Verification items for the finished model (mm, model axes). Face numbers are marked on the shaded views. A direction names the side the tool comes from. Round coordinates to 2 decimals unless told otherwise and drop trailing zeros. Write each loop counter-clockwise with the first axis right and the second up, starting at its lowest first coordinate (ties: lowest second). Pieces come first, ordered by that corner, then holes.
from build123d import *

# Parameters (mm, degrees)
EXTRUDE_1_DEPTH     = 34
SKETCH_2_R          = 2.75
CUT_EXTRUDE_1_DEPTH = 43.95346319
SKETCH_3_R          = 2.75
CUT_EXTRUDE_2_DEPTH = 45.226688775


with BuildPart() as part:
    # ｽｹｯﾁ1 → ﾎﾞｽ - 押し出し1 (new body)
    with BuildSketch(Plane.XY):
        Polygon((0, 0), (17, 0), (17, 17), (20, 17), (20, -3), (0, -3), align=None)
    extrude(amount=EXTRUDE_1_DEPTH)

    # ｽｹｯﾁ2 → ｶｯﾄ - 押し出し1 (cut, through all)
    with BuildSketch(Plane(origin=(20, 0, 0), x_dir=(0, 0, -1), z_dir=(1, 0, 0))):
        with Locations((-27, 7)):
            Circle(SKETCH_2_R)
        with Locations((-7, 7)):
            Circle(SKETCH_2_R)
    extrude(amount=-CUT_EXTRUDE_1_DEPTH, mode=Mode.SUBTRACT)

    # ｽｹｯﾁ3 → ｶｯﾄ - 押し出し2 (cut, through all)
    with BuildSketch(Plane.XZ.offset(3)):
        with Locations(Location((5, 7, 0), (0, 0, 270))):
            Circle(SKETCH_3_R)
        with Locations(Location((5, 27, 0), (0, 0, 270))):
            Circle(SKETCH_3_R)
    extrude(amount=-CUT_EXTRUDE_2_DEPTH, mode=Mode.SUBTRACT)


solid = part.part
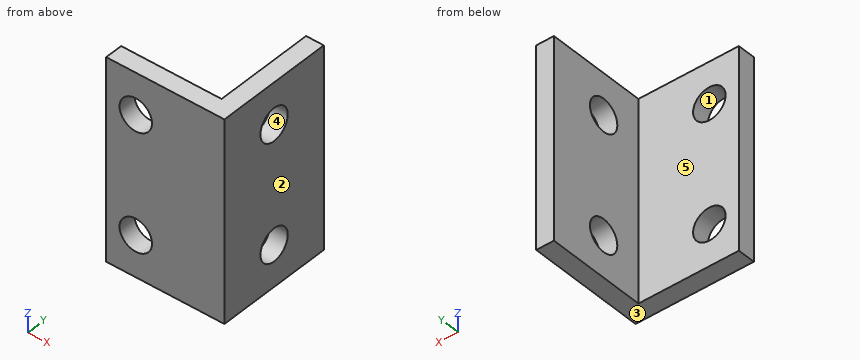
Q1. Material ranges on line 1 along Z through (x, y) = (7, -1.75); line 2 along X through (y, z) = (-2.15, 27); line 3 along X through (y, z) = (9, 11), recorded low to high.
Recorded:
line 1: z = 0 to 5.11, 8.89 to 25.11, 28.89 to 34
line 2: x = 0 to 2.25, 7.75 to 20
line 3: x = 17 to 20
Q2. Sectioned sample at A-A (y = 7). Enter the section's corners in (x, z).
Recorded:
outline: (17, 0) - (20, 0) - (20, 4.25) - (17, 4.25) - close; (17, 9.75) - (20, 9.75) - (20, 24.25) - (17, 24.25) - close; (17, 29.75) - (20, 29.75) - (20, 34) - (17, 34) - close
Q3. Sectioned sample at D-D (z = 12). Enter the section's corners in (x, y).
Recorded:
outline: (0, -3) - (20, -3) - (20, 17) - (17, 17) - (17, 0) - (0, 0) - close
Q4. Sectioned sample at B-B (x = 5). Enter the section's corners in (y, z), plus the area to 3 significant figures.
Recorded:
outline: (-3, 0) - (0, 0) - (0, 4.25) - (-3, 4.25) - close; (-3, 9.75) - (0, 9.75) - (0, 24.25) - (-3, 24.25) - close; (-3, 29.75) - (0, 29.75) - (0, 34) - (-3, 34) - close
area: 69.0 mm2
Q5. Release check for a two-part mould opening along Z. For the marked faces 1, 2 and 3 record: released by +Z, released by -Z, zero draft, split by the parting line, or undercut.
Recorded:
face 1: undercut
face 2: zero draft
face 3: released by -Z
Q6. Tool access check on the marked faces 4 and 5. Record the directions out of +Z, -Z, +X, -X, +Y, -Y that give a thin tool (end or side, any length) a straight path to the whole face; none if there is none.
Recorded:
face 4: +X, -X
face 5: +Z, -Z, -X, +Y
Q7. Depth check by flat-ended pin: P1, Ø6, axis at y = 8, z = 23.5, coming from the -X side; P2, Ø5, axis at x = 8, z = 18.5, coming from the +Y side; P3, Ø9, axis at y = 7, z = 27, coming from the +X side. Enter the tip coordinate at first touch or a pass-through.
Recorded:
P1: stops at x = 17
P2: stops at y = 0
P3: stops at x = 20
Q8. Sectioned sample at C-C (z = 27). Enter the section's corners in (x, y).
Recorded:
outline: (0, -3) - (2.25, -3) - (2.25, 0) - (0, 0) - close; (7.75, -3) - (20, -3) - (20, 4.25) - (17, 4.25) - (17, 0) - (7.75, 0) - close; (17, 9.75) - (20, 9.75) - (20, 17) - (17, 17) - close
